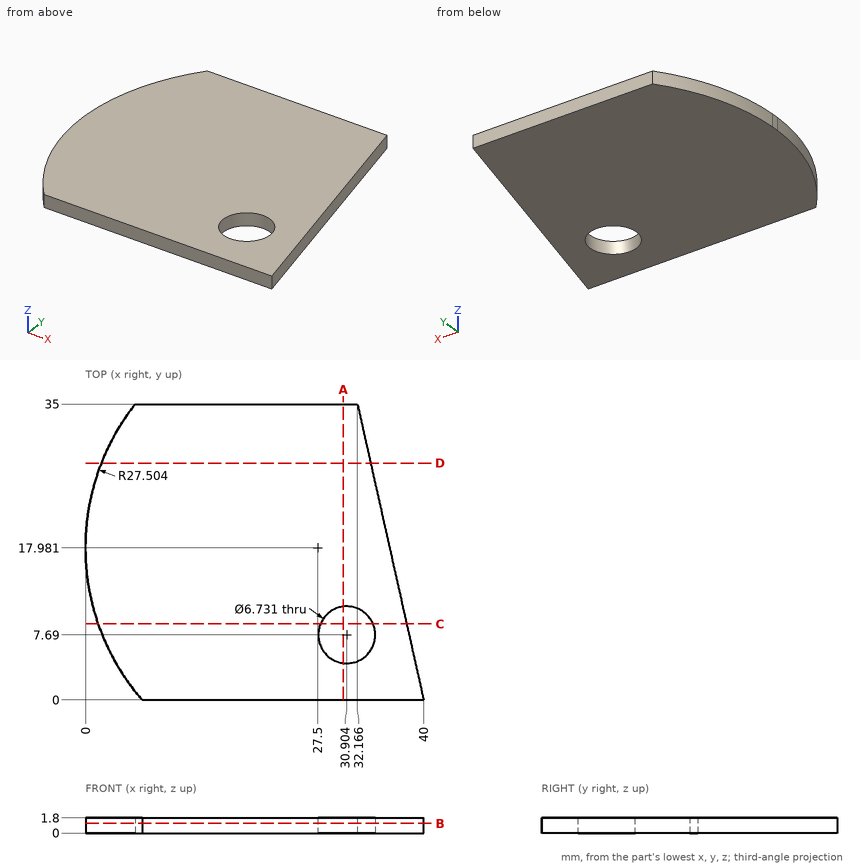
Job drawing, mm, ordinate dimensions from the low corner. One solid piece. Give positions to 0.01 mm unless a question says otherwise; leave off trailing zeros. Loops run counter-clockwise (first coordinate to the right, second up) from the corner with the lowest first, then second, coordinate; pieces in that order, holes last. Notation, with made-up numbers: M -7,87 L 3,87 A32 cw 3,114 Z; hole C 72,55.25 d7. An arc over 180 degrees is marked long. Put each result on its own line as item: value. Start each with the question number.
1) Saw through at A-A (x = 30.5). List the corners of the cut face in (y, z).
2) Flat gauge pins, fed straight in: pin 1 (1 mm diameter, centred on y = 20.5, z = 0.5, fed in from -X); pin 2 (1 mm diameter, centred on y = 9.5, z = 0.5, fed in from +X) (1 decimal). Where does each tip first touch, or does it go through?
3) Saw through at D-D (y = 28). List the corners of the cut face in (x, z) (1 decimal).
4) Probe probe 1 along Y at (x, z) = (30.5, 0.1); probe 2 along X at (y, z) = (18.5, 0.55); probe 3 along X at (y, z) = (17, 1.5) (1 decimal). List the from-to ranges inside material, lowest first.
5) Saw through at B-B (z = 1.15). List the corners of the cut face in (x, y) (1 decimal), then the cut area to 3 significant figures.
6) Saw through at C-C (y = 9). List the corners of the cut face in (x, z) (1 decimal).
Numbers:
1. outline: M 0,0 L 4.35,0 L 4.35,1.8 L 0,1.8 Z; M 11.03,0 L 35,0 L 35,1.8 L 11.03,1.8 Z
2. pin 1: x = 0.07
2. pin 2: x = 38
3. outline: M 1.9,0 L 33.7,0 L 33.7,1.8 L 1.9,1.8 Z
4. probe 1: 0 to 4.35, 11.03 to 35
4. probe 2: 0 to 35.86
4. probe 3: 0 to 36.2
5. outline: M 0,17.5 A27.5 ccw 6.7,0 L 40,0 L 32.2,35 L 5.9,35 A27.5 ccw 0,18.5 Z; hole C 30.9,7.7 d6.7
5. area: 1,160 mm^2
6. outline: M 1.5,0 L 27.8,0 L 27.8,1.8 L 1.5,1.8 Z; M 34,0 L 38,0 L 38,1.8 L 34,1.8 Z
